from build123d import *

# Parameters (mm, degrees)
SKETCH1_W                                    = 55
SKETCH1_H                                    = 47
EXTRUDE1_DEPTH                               = 10
SKETCH2_R                                    = 23
EXTRUDE2_DEPTH                               = 8
SKETCH3_R                                    = 1.2
EXTRUDE3_DEPTH                               = 6
SKETCH4_R                                    = 1.2
EXTRUDE4_DEPTH                               = 6
SKETCH5_R                                    = 2.75
SKETCH5_R_2                                  = 1.65
EXTRUDE5_DEPTH                               = 1.5
SKETCH6_R                                    = 1.65
EXTRUDE6_DEPTH                               = 2
SKETCH7_R                                    = 3.635
EXTRUDE7_DEPTH                               = 3
CSK_FOR_M1_6_COUNTERSUNK_FLAT_HEAD_S_2_COUNT = 2
CSK_FOR_M1_6_COUNTERSUNK_FLAT_HEAD_S_2_PITCH = 10.41
CSK_FOR_M1_6_COUNTERSUNK_FLAT_HEAD_S_3_COUNT = 2
CSK_FOR_M1_6_COUNTERSUNK_FLAT_HEAD_S_3_PITCH = 10.409719016
CHAMFER1_SIZE                                = 1.8
CHAMFER1_SIZE2                               = 3.117691454
F_3_4_3_4_DIAMETER_HOLE1_D                   = 3.4
F_3_4_3_4_DIAMETER_HOLE1_DEPTH               = 4
F_3_4_3_4_DIAMETER_HOLE1_TIP                 = 1.021463052


with BuildPart() as part:
    # Sketch1 → Extrude1 (new body)
    with BuildSketch(Plane(origin=(0, 0, 0), x_dir=(0, 0, -1), z_dir=(1, 0, 0))):
        with Locations((-14.681315866, 9.625451264)):
            Rectangle(SKETCH1_W, SKETCH1_H)
    extrude(amount=EXTRUDE1_DEPTH)

    # Sketch2 → Extrude2 (cut)
    with BuildSketch(Plane(origin=(10, 0, 0), x_dir=(0, 0, -1), z_dir=(1, 0, 0))):
        with Locations((-14.681315866, 5.625451264)):
            Circle(SKETCH2_R)
    extrude(amount=-EXTRUDE2_DEPTH, mode=Mode.SUBTRACT)

    # Sketch3 → Extrude3 (cut)
    with BuildSketch(Plane.XY.offset(42.181315866)):
        with Locations((5, 25.125451264)):
            Circle(SKETCH3_R)
        with Locations((7, -11.374548736)):
            Circle(SKETCH3_R)
    extrude(amount=-EXTRUDE3_DEPTH, mode=Mode.SUBTRACT)

    # Sketch4 → Extrude4 (cut)
    with BuildSketch(Plane(origin=(0, 0, -12.818684134), x_dir=(-1, 0, 0), z_dir=(0, 0, -1))):
        with Locations((-5, 25.125451264)):
            Circle(SKETCH4_R)
        with Locations((-7, -11.374548736)):
            Circle(SKETCH4_R)
    extrude(amount=-EXTRUDE4_DEPTH, mode=Mode.SUBTRACT)

    # Sketch5 → Extrude5 (add)
    with BuildSketch(Plane(origin=(2, 0, 0), x_dir=(0, 0, -1), z_dir=(1, 0, 0))):
        with Locations((-14.681315866, 5.625451264)):
            Circle(SKETCH5_R)
        with Locations((-14.681315866, 5.625451264)):
            Circle(SKETCH5_R_2, mode=Mode.SUBTRACT)
    extrude(amount=EXTRUDE5_DEPTH)

    # Sketch6 → Extrude6 (cut)
    with BuildSketch(Plane(origin=(2, 0, 0), x_dir=(0, 0, -1), z_dir=(1, 0, 0))):
        with Locations((-14.681315866, 5.625451264)):
            Circle(SKETCH6_R)
    extrude(amount=-EXTRUDE6_DEPTH, mode=Mode.SUBTRACT)

    # Sketch7 → Extrude7 (cut)
    with BuildSketch(Plane.ZY):
        with Locations((0.501315866, -0.554548736)):
            Circle(SKETCH7_R)
    extrude(amount=-EXTRUDE7_DEPTH, mode=Mode.SUBTRACT)

    # Sketch10 → CSK for M1.6 Countersunk Flat Head Screw1 (revolve, cut)
    with BuildSketch(Plane(origin=(2, 2.450451264, 5.706315866), x_dir=(0, 0, -1), z_dir=(0, 1, 0))):
        Polygon((0, 0), (0, 2), (1.025, 2), (1.025, 1.125), (2.15, 0), align=None)
    csk_for_m1_6_countersunk_flat_head_screw = revolve(axis=Axis((8.35, 2.450451264, 5.706315866), (-1, 0, 0)), mode=Mode.SUBTRACT)

    # CSK for M1.6 Countersunk Flat Head S 2: CSK for M1.6 Countersunk Flat Head Screw1 ×2
    with Locations(*[(0, 0, -i * CSK_FOR_M1_6_COUNTERSUNK_FLAT_HEAD_S_2_PITCH) for i in range(1, CSK_FOR_M1_6_COUNTERSUNK_FLAT_HEAD_S_2_COUNT)]):
        add(csk_for_m1_6_countersunk_flat_head_screw, mode=Mode.SUBTRACT)

    # CSK for M1.6 Countersunk Flat Head S 3: CSK for M1.6 Countersunk Flat Head Screw1 ×2
    with Locations(*[Vector(0, -0.866017612, -0.500013496) * (i * CSK_FOR_M1_6_COUNTERSUNK_FLAT_HEAD_S_3_PITCH) for i in range(1, CSK_FOR_M1_6_COUNTERSUNK_FLAT_HEAD_S_3_COUNT)]):
        add(csk_for_m1_6_countersunk_flat_head_screw, mode=Mode.SUBTRACT)

    # Chamfer1
    chamfer1_edges = [part.edges().sort_by_distance(p)[0] for p in [
        (0, 9.625451264, -12.818684134),
        (0, 9.625451264, 42.181315866),
    ]]
    chamfer1_side = [part.faces().sort_by_distance(p)[0] for p in [
        (0, 9.84627635, 14.970036249),
    ]]
    chamfer(chamfer1_edges, length=CHAMFER1_SIZE, length2=CHAMFER1_SIZE2, reference=chamfer1_side[0])

    # Ø3.4 (3.4) Diameter Hole1
    with Locations(Plane(origin=(5, 33.125451264, -7.318684134), x_dir=(0, 0, 1), z_dir=(0, 1, 0))):
        with Locations((0, 0), (44, 0)):
            Hole(F_3_4_3_4_DIAMETER_HOLE1_D / 2, depth=F_3_4_3_4_DIAMETER_HOLE1_DEPTH)
            with Locations((0, 0, -(F_3_4_3_4_DIAMETER_HOLE1_DEPTH + F_3_4_3_4_DIAMETER_HOLE1_TIP / 2))):  # 118° drill point
                Cone(0, F_3_4_3_4_DIAMETER_HOLE1_D / 2, F_3_4_3_4_DIAMETER_HOLE1_TIP, mode=Mode.SUBTRACT)


solid = part.part
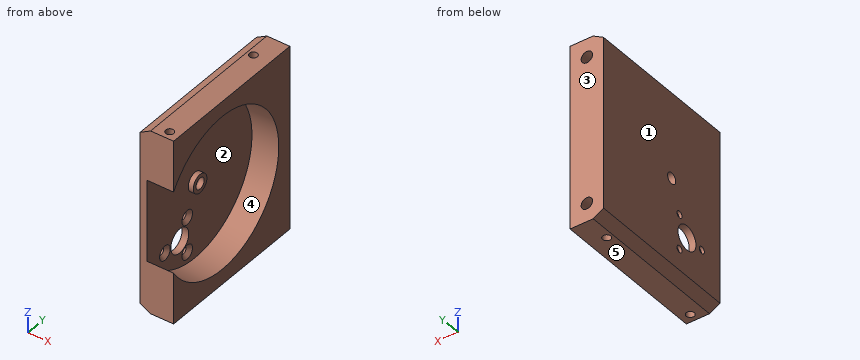
Can you work these out from the model? Positions are in its coordinate system, mm. Face numbers are marked on the shaded views. A direction names the side the tool comes from. Round coordinates to 2 decimals unless told otherwise and drop trailing zeros. Loops run counter-clockwise (first coordinate to the right, second up) from the corner with the lowest first, then second, coordinate; pieces in that order, holes last. Notation, with made-up numbers: (80, 46.25) - (116, 46.25) arc R19 cw to (116, 62.25) - close; hole circle Ø3 at (19, 5.5). An arc over 180 degrees is marked (long way). Write item = value, one per line. Start each with the question number.
(1) If we section it at B-B (z = 33.5): Please give me the cut outline in (x, y), and give its area (3 significant figures).
(2) If we section it at A-A (x = 9.25): Please give me the cut outline in (y, z) (3 decimals), and give its area (3 significant figures).
(3) For the marked faces 4 and 5, which set-ups out of +Z, -Z, +X, -X, +Y, -Y let a thin tool reach every point of the face, with its end or its side?
(4) For P1, Ø6, axis at y = 6, z = 13.5, coming from the +X side; P2, Ø4, axis at x = 5, y = 25.13, coming from the -Z side; P3, Ø2, axis at x = 5, z = 23, coming from the -Y side; P4, Ø1.9, axis at x = 7, y = -11.5, coming from the -Z side, each with a flat end and sliding along its axis, tell me the tip position at first contact or that it passes through.
(5) If I drill on probe 1 along Z at (x, y) = (5, 31.2); probe 2 along Y at (x, z) = (3.25, 14); probe 3 along X at (y, z) = (-3.5, 14.5), over which ranges is the centre line in solid material (lowest first)? Write a range as [from, to].
(6) If we mould it in two halves opening along Y, with no side actions, what happens to the marked faces 1, 2 and 3? For each: released by +Y, released by -Y, zero draft, split by the parting line, or undercut.
Ans:
q1.outline = (0, -13.87) - (10, -13.87) - (10, -7.6) - (2, -7.6) - (2, 18.85) - (10, 18.85) - (10, 33.13) - (0, 33.13) - close
q1.area = 258 mm²
q2.outline = (-13.875, -12.819) - (33.125, -12.819) - (33.125, 42.181) - (-13.875, 42.181) - (-13.875, 26.878) arc R23 cw (long way) to (-13.875, 2.485) - close
q2.area = 981 mm²
q3.face_4 = +X
q3.face_5 = -Z, +X, -X, +Y, -Y
q4.P1 = 3.5
q4.P2 = -12.82
q4.P3 = 26.65
q4.P4 = -6.82
q5.probe_1 = [-12.82, -9.02], [-5.62, 34.98], [38.38, 42.18]
q5.probe_2 = [2.96, 4.12], [7.13, 8.29], [28.62, 33.13]
q5.probe_3 = [0, 2]
q6.face_1 = zero draft
q6.face_2 = undercut
q6.face_3 = released by +Y
